```python
from build123d import *

# Parameters (mm, degrees)
F0_W         = 80
F0_H         = 60
F1_DEPTH     = 130
F2_T         = -1.5
F3_W         = 1.5
F3_H         = 27
F4_DEPTH     = 91
F5_R         = 1
F6_W         = 17
F6_H         = 16
F6_W_2       = 1.5
F6_H_2       = 27
F7_DEPTH     = 2
F8_T1_DEPTH  = 92
F8_T3_DEPTH  = 29.9726896882
F8_S7_W      = 1
F8_S7_H      = 1
F8_T8_DEPTH  = 1
F8_T15_DEPTH = 29.9726896882
F8_T19_DEPTH = 94.5
F9_T1_DEPTH  = 127.5
F9_T3_DEPTH  = 58.5
F9_S7_W      = 1
F9_S7_H      = 1
F9_T8_DEPTH  = 1
F9_S13_W     = 1
F9_S13_H     = 1
F9_T14_DEPTH = 1
F9_T18_ANGLE = 90
F11_DEPTH    = 60
F12_DEPTH    = 60
F13_DEPTH    = 50
F14_R        = 2
F15_W        = 17
F15_H        = 16
F16_DEPTH    = 91


# Not quite as in the source:
# - a fillet or chamfer that OpenCascade refuses, or shapes differently, is made with other operations: its cross-section is extruded or revolved along the edge and cut away or added


with BuildPart() as f1:
    # F0 (on Top) → F1 (new body)
    with BuildSketch(Plane.XY):
        Rectangle(F0_W, F0_H)
    extrude(amount=F1_DEPTH)

    # F2
    f2_openings = [f1.faces().sort_by_distance(p)[0] for p in [
        (0, 0, 130),
    ]]
    offset(amount=F2_T, openings=f2_openings)

    # F3 (on face) → F4 (join)
    with BuildSketch(Plane.XY.offset(1.5)):
        with Locations((11.75, -15)):
            Rectangle(F3_W, F3_H)
    extrude(amount=F4_DEPTH)

    # F5
    f5_edges = [f1.edges().sort_by_distance(p)[0] for p in [
        (0, 28.5, 1.5),
        (-38.5, 0, 1.5),
        (-13.75, -28.5, 1.5),
        (11, -15, 1.5),
    ]]
    fillet(f5_edges, radius=F5_R)

    # F6 (on face) → F7 (join)
    with BuildSketch(Plane.XY.offset(92.5)):
        Polygon((38.4726896882, -1.5), (12.5, -1.5), (12.5, -28.5), (11, -28.5), (11, -28.532365337), (38.4726896882, -28.532365337), align=None)
        with Locations((24.7363448441, -15)):
            Rectangle(F6_W, F6_H, mode=Mode.SUBTRACT)
        with Locations((11.75, -15)):
            Rectangle(F6_W_2, F6_H_2)
    extrude(amount=F7_DEPTH)

    # F8: fillet of radius 1 on 2 edges, made by hand

    # F8_s2 → F8_t1 (join)
    with BuildSketch(Plane.XY.offset(2.5)):
        with BuildLine():
            ThreePointArc((10, -28.5), (10.7071067812, -28.2071067812), (11, -27.5))
            Line((11, -27.5), (11, -28.5))
            Line((11, -28.5), (10, -28.5))
        make_face()
    extrude(amount=F8_T1_DEPTH)

    # F8_s4 → F8_t3 (join)
    with BuildSketch(Plane.YZ.offset(11)):
        with BuildLine():
            ThreePointArc((-28.5, 95.5), (-28.2071067812, 94.7928932188), (-27.5, 94.5))
            Line((-27.5, 94.5), (-28.5, 94.5))
            Line((-28.5, 94.5), (-28.5, 95.5))
        make_face()
    extrude(amount=F8_T3_DEPTH)


with BuildPart() as f8_tool6:
    # F8_s7 → F8_t8 (new body)
    with BuildSketch(Plane.XZ.offset(27.5)):
        with Locations((10.5, 2)):
            Rectangle(F8_S7_W, F8_S7_H)
    extrude(amount=F8_T8_DEPTH)

    # F8_s9 → F8_t10 (revolve, cut)
    with BuildSketch(Plane(origin=(10, -27.5, 2.5), x_dir=(-0.7071067812, 0, 0.7071067812), z_dir=(0.7071067812, 0, 0.7071067812))):
        with BuildLine():
            ThreePointArc((0, -1), (1, 0), (0, 1))
            Line((0, 1), (0, -1))
        make_face()
    revolve(axis=Axis((10, -27.5, 2.5), (0, -1, 0)), mode=Mode.SUBTRACT)


with BuildPart() as f1_1:
    add(f1.part)

    # F8_t5: union F8_tool6
    add(f8_tool6.part)


with BuildPart() as f8_tool13:
    # F8_s14 → F8_t15 (new body)
    with BuildSketch(Plane.YZ.offset(8.5)):
        with BuildLine():
            ThreePointArc((-28.5, 95.5), (-28.2071067812, 94.7928932188), (-27.5, 94.5))
            Line((-27.5, 94.5), (-28.5, 94.5))
            Line((-28.5, 94.5), (-28.5, 95.5))
        make_face()
    extrude(amount=F8_T15_DEPTH)

    split(bisect_by=Plane.YZ.offset(11), keep=Keep.BOTTOM)


with BuildPart() as f8_tool17:
    # F8_s18 → F8_t19 (new body)
    with BuildSketch(Plane.XY.offset(97)):
        with BuildLine():
            ThreePointArc((10, -28.5), (10.7071067812, -28.2071067812), (11, -27.5))
            Line((11, -27.5), (11, -28.5))
            Line((11, -28.5), (10, -28.5))
        make_face()
    extrude(amount=-F8_T19_DEPTH)

    split(bisect_by=Plane.XY.offset(94.5), keep=Keep.TOP)


with BuildPart() as f8_tool13_1:
    add(f8_tool13.part)

    # F8_t21: intersect F8_tool17
    add(f8_tool17.part, mode=Mode.INTERSECT)


with BuildPart() as f1_2:
    add(f1_1.part)

    # F8_t11: union F8_tool13
    add(f8_tool13_1.part)

    # F9: fillet of radius 1 on 3 edges, made by hand

    # F9_s2 → F9_t1 (join)
    with BuildSketch(Plane.XY.offset(2.5)):
        with BuildLine():
            ThreePointArc((-37.5, -28.5), (-38.2071067812, -28.2071067812), (-38.5, -27.5))
            Line((-38.5, -27.5), (-38.5, -28.5))
            Line((-38.5, -28.5), (-37.5, -28.5))
        make_face()
        with BuildLine():
            ThreePointArc((-37.5, 28.5), (-38.2071067812, 28.2071067812), (-38.5, 27.5))
            Line((-38.5, 27.5), (-38.5, 28.5))
            Line((-38.5, 28.5), (-37.5, 28.5))
        make_face()
        with BuildLine():
            ThreePointArc((37.5, 28.5), (38.2071067812, 28.2071067812), (38.5, 27.5))
            Line((38.5, 27.5), (38.5, 28.5))
            Line((38.5, 28.5), (37.5, 28.5))
        make_face()
    extrude(amount=F9_T1_DEPTH)

    # F9_s4 → F9_t3 (join)
    with BuildSketch(Plane.XZ.offset(-27.5)):
        with BuildLine():
            ThreePointArc((38.5, 2.5), (38.2071067812, 1.7928932188), (37.5, 1.5))
            Line((37.5, 1.5), (38.5, 1.5))
            Line((38.5, 1.5), (38.5, 2.5))
        make_face()
    extrude(amount=F9_T3_DEPTH)


with BuildPart() as f9_tool6:
    # F9_s7 → F9_t8 (new body)
    with BuildSketch(Plane.XZ.offset(-27.5)):
        with Locations((-38, 2)):
            Rectangle(F9_S7_W, F9_S7_H)
    extrude(amount=-F9_T8_DEPTH)

    # F9_s9 → F9_t10 (revolve, cut)
    with BuildSketch(Plane(origin=(-37.5, 27.5, 2.5), x_dir=(0.7071067812, 0, 0.7071067812), z_dir=(-0.7071067812, 0, 0.7071067812))):
        with BuildLine():
            ThreePointArc((0, -1), (1, 0), (0, 1))
            Line((0, 1), (0, -1))
        make_face()
    revolve(axis=Axis((-37.5, 27.5, 2.5), (0, 1, 0)), mode=Mode.SUBTRACT)


with BuildPart() as f1_3:
    add(f1_2.part)

    # F9_t5: union F9_tool6
    add(f9_tool6.part)


with BuildPart() as f9_tool12:
    # F9_s13 → F9_t14 (new body)
    with BuildSketch(Plane.XZ.offset(27.5)):
        with Locations((-38, 2)):
            Rectangle(F9_S13_W, F9_S13_H)
    extrude(amount=F9_T14_DEPTH)

    # F9_s15 → F9_t16 (revolve, cut)
    with BuildSketch(Plane(origin=(-37.5, -27.5, 2.5), x_dir=(0.7071067812, 0, 0.7071067812), z_dir=(0.7071067812, 0, -0.7071067812))):
        with BuildLine():
            ThreePointArc((0, -1), (1, 0), (0, 1))
            Line((0, 1), (0, -1))
        make_face()
    revolve(axis=Axis((-37.5, -27.5, 2.5), (0, -1, 0)), mode=Mode.SUBTRACT)


with BuildPart() as f1_4:
    add(f1_3.part)

    # F9_t11: union F9_tool12
    add(f9_tool12.part)

    # F9_s17 → F9_t18 (revolve)
    with BuildSketch(Plane.XY.offset(2.5)):
        with BuildLine():
            ThreePointArc((38.5, 27.5), (38.2071067812, 28.2071067812), (37.5, 28.5))
            Line((37.5, 28.5), (38.5, 28.5))
            Line((38.5, 28.5), (38.5, 27.5))
        make_face()
    revolve(axis=Axis((38.5, 27.5, 2.5), (-1, 0, 0)), revolution_arc=F9_T18_ANGLE)

    # F10 (on face) → F11 (join)
    with BuildSketch(Plane(origin=(0, 30, 0), x_dir=(-1, 0, 0), z_dir=(0, 1, 0))):
        Polygon((-42.6013286531, 4), (-41.4004783891, 2.4006374993), (-42.6, 1.5), (-44.4770764343, 4), (-45, 4), (-45, 0), (-40, 0), (-40, 4), align=None)
    extrude(amount=-F11_DEPTH)

    # F10 (on face) → F12 (join)
    with BuildSketch(Plane(origin=(0, 30, 0), x_dir=(-1, 0, 0), z_dir=(0, 1, 0))):
        Polygon((-65.4174783693, 34.3878804557), (-64.0949453732, 32.6264537871), (-40, 32.6264537871), (-40, 35.6264537871), (-68, 35.6264537871), (-68, 32.6264537871), (-65.9706931543, 32.6264537871), (-66.6169999802, 33.4872429564), align=None)
    extrude(amount=-F12_DEPTH)

    # F14
    f14_edges = [f1_4.edges().sort_by_distance(p)[0] for p in [
        (40, 0, 35.626454),
        (40, 0, 4),
        (40, 0, 32.626454),
    ]]
    fillet(f14_edges, radius=F14_R)


with BuildPart() as f13:
    # F10 (on face) → F13 (new body)
    with BuildSketch(Plane(origin=(0, 30, 0), x_dir=(-1, 0, 0), z_dir=(0, 1, 0))):
        Polygon((-42.6, 1.5), (-41.4004783891, 2.4006374993), (-42.6013286531, 4), (-44.4770764343, 4), align=None)
        Polygon((-44.4770764343, 4), (-42.6013286531, 4), (-64.0949453732, 32.6264537871), (-65.9706931543, 32.6264537871), align=None)
        Polygon((-65.9706931543, 32.6264537871), (-64.0949453732, 32.6264537871), (-65.4174783693, 34.3878804557), (-66.6169999802, 33.4872429564), align=None)
    extrude(amount=-F13_DEPTH)


with BuildPart() as f16:
    # F15 (on face) → F16 (new body)
    with BuildSketch(Plane(origin=(0, 0, 92.5), x_dir=(1, 0, 0), z_dir=(0, 0, -1))):
        with BuildLine():
            ThreePointArc((12.5, 6.589983932), (14.2478802784, 3.7576947486), (17.3863448441, 2.65))
            Line((17.3863448441, 2.65), (32.0863448441, 2.65))
            ThreePointArc((32.0863448441, 2.65), (35.62187875, 4.1144660941), (37.0863448441, 7.65))
            Line((37.0863448441, 7.65), (37.0863448441, 22.35))
            ThreePointArc((37.0863448441, 22.35), (35.62187875, 25.8855339059), (32.0863448441, 27.35))
            Line((32.0863448441, 27.35), (17.3863448441, 27.35))
            ThreePointArc((17.3863448441, 27.35), (14.2478802784, 26.2423052514), (12.5, 23.410016068))
            Line((12.5, 23.410016068), (12.5, 6.589983932))
        make_face()
        with Locations((24.7363448441, 15)):
            Rectangle(F15_W, F15_H, mode=Mode.SUBTRACT)
        with Locations((24.7363448441, 15)):
            Rectangle(F15_W, F15_H)
    extrude(amount=F16_DEPTH)


solid = f16.part
```
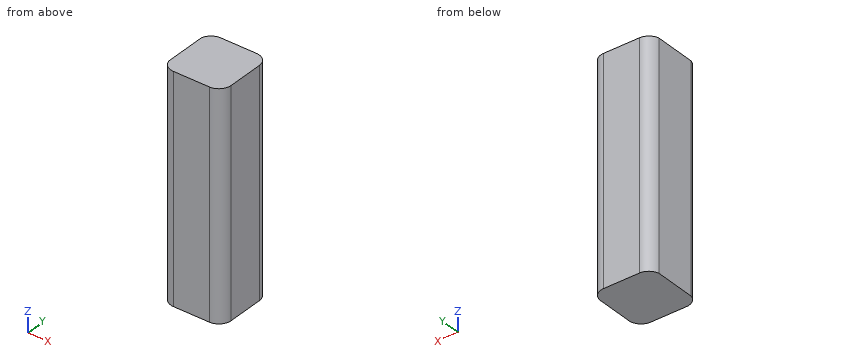
The model under review builds one solid part; all positions refer to its coordinate system, in mm. Round coordinates to 2 decimals unless told otherwise and drop trailing zeros. Order: outer loops, then holes, each group sorted by start corner. A loop starts at its lowest first (then second) coordinate and runs counter-clockwise, first axis right, second up. Notation, with made-up numbers: (73.5, -38.75) -> (95.5, -38.75) arc R27 ccw to (95.5, -12.75) -> close; hole circle Ø6 at (-8.5, 13.25). An arc over 180 degrees is marked (long way). One line per item, written item: value. Start each with the question number.
Q1. Take a section at C-C (x = 34.25). Write out the cut boundary in (y, z), and give its area (3 significant figures).
Q2. Take a section at B-B (y = -24.5). Write out the cut boundary in (x, z), and give its area (3 significant figures).
Q3. Wall thickness on line 1 (Y direction, x = 17.25, z = 60); line 2 (X direction, y = -6, z = 42); line 3 (Y direction, x = 16.25, z = 60): over which ranges is each line inside the solid? List them lowest first.
Q4. Take a section at A-A (z = 71.5). Write out the cut boundary in (x, y).
Reported:
1. outline: (-26.86, 1.5) -> (-3.14, 1.5) -> (-3.14, 92.5) -> (-26.86, 92.5) -> close
1. area: 2,160 mm2
2. outline: (12.87, 1.5) -> (36.6, 1.5) -> (36.6, 92.5) -> (12.87, 92.5) -> close
2. area: 2,160 mm2
3. line 1: y = -27.35 to -2.65
3. line 2: x = 12.67 to 36.81
3. line 3: y = -27.22 to -2.78
4. outline: (12.5, -23.41) arc R5 ccw to (17.39, -27.35) -> (32.09, -27.35) arc R5 ccw to (37.09, -22.35) -> (37.09, -7.65) arc R5 ccw to (32.09, -2.65) -> (17.39, -2.65) arc R5 ccw to (12.5, -6.59) -> close
